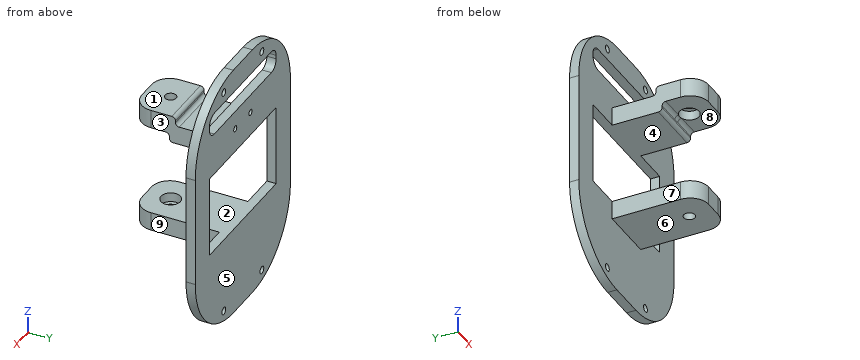
```python
from build123d import *

# Parameters (mm, degrees)
SKETCH1_W           = 100
SKETCH1_H           = 90
BOSS_EXTRUDE1_DEPTH = 5
SKETCH2_W           = 70
SKETCH2_H           = 44
CUT_EXTRUDE1_DEPTH  = 68.453687816
SKETCH3_R           = 1.6
CUT_EXTRUDE2_DEPTH  = 68.453687816
SKETCH4_W           = 100
SKETCH4_H           = 25
BOSS_EXTRUDE2_DEPTH = 5
SKETCH6_W           = 70
SKETCH6_H           = 12
CUT_EXTRUDE4_DEPTH  = 17
SKETCH8_W           = 30
SKETCH8_H           = 10
BOSS_EXTRUDE4_DEPTH = 47
SKETCH11_R          = 5.25
CUT_EXTRUDE5_DEPTH  = 5
SKETCH12_R          = 3
CUT_EXTRUDE6_DEPTH  = 5
FILLET1_R           = 10
CUT_EXTRUDE7_START  = -5
SKETCH13_R          = 5.25
CUT_EXTRUDE7_DEPTH  = 5
CUT_EXTRUDE8_START  = -5
SKETCH14_R          = 3
CUT_EXTRUDE8_DEPTH  = 5
FILLET2_R           = 10
SKETCH15_R          = 2
CUT_EXTRUDE9_DEPTH  = 101.518654985
FILLET3_R           = 40
FILLET4_R           = 40
FILLET5_R           = 5
BOSS_EXTRUDE5_DEPTH = 30
SKETCH17_R          = 5.25
CUT_EXTRUDE10_DEPTH = 10
SKETCH18_R          = 3
CUT_EXTRUDE12_DEPTH = 21
CUT_EXTRUDE13_DEPTH = 21
SKETCH20_W          = 5
SKETCH20_H          = 20
CUT_EXTRUDE14_DEPTH = 107.46126056
FILLET6_R           = 2
FILLET7_R           = 2


with BuildPart() as part:
    # Sketch1 → Boss-Extrude1 (new body)
    with BuildSketch(Plane(origin=(0, 0, 0), x_dir=(1, 0, 0), z_dir=(0, 1, 0))):
        Rectangle(SKETCH1_W, SKETCH1_H)
    extrude(amount=BOSS_EXTRUDE1_DEPTH)

    # Sketch2 → Cut-Extrude1 (cut, through all)
    with BuildSketch(Plane(origin=(0, 5, 0), x_dir=(1, 0, 0), z_dir=(0, 1, 0))):
        Rectangle(SKETCH2_W, SKETCH2_H)
    extrude(amount=-CUT_EXTRUDE1_DEPTH, mode=Mode.SUBTRACT)

    # Sketch3 → Cut-Extrude2 (cut, through all)
    with BuildSketch(Plane(origin=(0, 5, 0), x_dir=(1, 0, 0), z_dir=(0, 1, 0))):
        with Locations(Location((-8, -35, 0), (0, 0, 270))):
            Circle(SKETCH3_R)
        with Locations(Location((8, -35, 0), (0, 0, 90))):
            Circle(SKETCH3_R)
    extrude(amount=-CUT_EXTRUDE2_DEPTH, mode=Mode.SUBTRACT)

    # Sketch4 → Boss-Extrude2 (add)
    with BuildSketch(Plane(origin=(0, 5, 0), x_dir=(1, 0, 0), z_dir=(0, 1, 0))):
        with Locations((0, -57.5)):
            Rectangle(SKETCH4_W, SKETCH4_H)
        with Locations((0, 57.5)):
            Rectangle(SKETCH4_W, SKETCH4_H)
    extrude(amount=-BOSS_EXTRUDE2_DEPTH)

    # Sketch6 → Cut-Extrude4 (cut)
    with BuildSketch(Plane(origin=(0, 5, 0), x_dir=(1, 0, 0), z_dir=(0, 1, 0))):
        with Locations((0, -51)):
            Rectangle(SKETCH6_W, SKETCH6_H)
    extrude(amount=-CUT_EXTRUDE4_DEPTH, mode=Mode.SUBTRACT)

    # Sketch8 → Boss-Extrude4 (add)
    with BuildSketch(Plane.XZ):
        with Locations((0, 27)):
            Rectangle(SKETCH8_W, SKETCH8_H)
        with Locations((0, -27)):
            Rectangle(SKETCH8_W, SKETCH8_H)
    extrude(amount=BOSS_EXTRUDE4_DEPTH)

    # Sketch11 → Cut-Extrude5 (cut)
    with BuildSketch(Plane(origin=(0, 0, 22), x_dir=(-1, 0, 0), z_dir=(0, 0, -1))):
        with Locations((0, -34)):
            Circle(SKETCH11_R)
    extrude(amount=-CUT_EXTRUDE5_DEPTH, mode=Mode.SUBTRACT)

    # Sketch12 → Cut-Extrude6 (cut)
    with BuildSketch(Plane(origin=(0, 0, 27), x_dir=(-1, 0, 0), z_dir=(0, 0, -1))):
        with Locations((0, -34)):
            Circle(SKETCH12_R)
    extrude(amount=-CUT_EXTRUDE6_DEPTH, mode=Mode.SUBTRACT)

    # Fillet1
    fillet1_edges = [part.edges().sort_by_distance(p)[0] for p in [
        (-15, -47, 27),
        (15, -47, 27),
    ]]
    fillet(fillet1_edges, radius=FILLET1_R)

    # Sketch13 → Cut-Extrude7 (cut)
    with BuildSketch(Plane.XY.offset(-22).offset(CUT_EXTRUDE7_START)):
        with Locations(Location((0, -34, 0), (0, 0, 180))):
            Circle(SKETCH13_R)
    extrude(amount=CUT_EXTRUDE7_DEPTH, mode=Mode.SUBTRACT)

    # Sketch14 → Cut-Extrude8 (cut)
    with BuildSketch(Plane.XY.offset(-27).offset(CUT_EXTRUDE8_START)):
        with Locations(Location((0, -34, 0), (0, 0, 180))):
            Circle(SKETCH14_R)
    extrude(amount=CUT_EXTRUDE8_DEPTH, mode=Mode.SUBTRACT)

    # Fillet2
    fillet2_edges = [part.edges().sort_by_distance(p)[0] for p in [
        (15, -47, -27),
        (-15, -47, -27),
    ]]
    fillet(fillet2_edges, radius=FILLET2_R)

    # Sketch15 → Cut-Extrude9 (cut, through all)
    with BuildSketch(Plane(origin=(0, 5, 0), x_dir=(1, 0, 0), z_dir=(0, 1, 0))):
        with Locations(Location((-20, -63, 0), (0, 0, 270))):
            Circle(SKETCH15_R)
        with Locations(Location((-20, 63, 0), (0, 0, 270))):
            Circle(SKETCH15_R)
        with Locations(Location((20, -63, 0), (0, 0, 270))):
            Circle(SKETCH15_R)
        with Locations(Location((20, 63, 0), (0, 0, 270))):
            Circle(SKETCH15_R)
    extrude(amount=-CUT_EXTRUDE9_DEPTH, mode=Mode.SUBTRACT)

    # Fillet3
    fillet3_edges = [part.edges().sort_by_distance(p)[0] for p in [
        (-50, 2.5, 70),
        (50, 2.5, 70),
    ]]
    fillet(fillet3_edges, radius=FILLET3_R)

    # Fillet4
    fillet4_edges = [part.edges().sort_by_distance(p)[0] for p in [
        (-50, 2.5, -70),
        (50, 2.5, -70),
    ]]
    fillet(fillet4_edges, radius=FILLET4_R)

    # Fillet5
    fillet5_edges = [part.edges().sort_by_distance(p)[0] for p in [
        (-35, 2.5, 57),
        (-35, 2.5, 45),
        (35, 2.5, 45),
        (35, 2.5, 57),
    ]]
    fillet(fillet5_edges, radius=FILLET5_R)

    # Sketch16 → Boss-Extrude5 (add)
    with BuildSketch(Plane(origin=(15, 0, 0), x_dir=(0, 0, -1), z_dir=(1, 0, 0))):
        Polygon((-32, -23.652392467), (-37, -23.652392467), (-37, -47), (-27, -47), (-27, -23.652392467), align=None)
    extrude(amount=-BOSS_EXTRUDE5_DEPTH)

    # Sketch17 → Cut-Extrude10 (cut)
    with BuildSketch(Plane(origin=(0, 0, 22), x_dir=(-1, 0, 0), z_dir=(0, 0, -1))):
        with Locations((0, -34)):
            Circle(SKETCH17_R)
    extrude(amount=-CUT_EXTRUDE10_DEPTH, mode=Mode.SUBTRACT)

    # Sketch18 → Cut-Extrude12 (cut)
    with BuildSketch(Plane(origin=(0, 0, 22), x_dir=(-1, 0, 0), z_dir=(0, 0, -1))):
        with Locations(Location((0, -34, 0), (0, 0, 180))):
            Circle(SKETCH18_R)
    extrude(amount=-CUT_EXTRUDE12_DEPTH, mode=Mode.SUBTRACT)

    # Sketch19 → Cut-Extrude13 (cut)
    with BuildSketch(Plane(origin=(0, 0, 22), x_dir=(-1, 0, 0), z_dir=(0, 0, -1))):
        with BuildLine():
            Line((-15, -37), (-15, -47))
            Line((-15, -47), (-5, -47))
            ThreePointArc((-5, -47), (-12.071067812, -44.071067812), (-15, -37))
        make_face()
        with BuildLine():
            Line((5, -47), (15, -47))
            Line((15, -47), (15, -37))
            ThreePointArc((15, -37), (12.071067812, -44.071067812), (5, -47))
        make_face()
    extrude(amount=-CUT_EXTRUDE13_DEPTH, mode=Mode.SUBTRACT)

    # Sketch20 → Cut-Extrude14 (cut, through all)
    with BuildSketch(Plane(origin=(15, 0, 0), x_dir=(0, 0, -1), z_dir=(1, 0, 0))):
        with Locations((-24.5, -37)):
            Rectangle(SKETCH20_W, SKETCH20_H)
    extrude(amount=-CUT_EXTRUDE14_DEPTH, mode=Mode.SUBTRACT)

    # Fillet6
    fillet6_edges = [part.edges().sort_by_distance(p)[0] for p in [
        (0, -23.652392467, 32),
        (0, -23.652392467, 37),
    ]]
    fillet(fillet6_edges, radius=FILLET6_R)

    # Fillet7
    fillet7_edges = [part.edges().sort_by_distance(p)[0] for p in [
        (0, -27, 27),
        (0, -27, 22),
    ]]
    fillet(fillet7_edges, radius=FILLET7_R)


solid = part.part
```
Work out the finished part from the listing and answer in its coordinate system (mm). Face numbers are marked on the shaded views. A direction names the side the tool comes from. Give positions to 0.01 mm unless a question says otherwise; leave off trailing zeros. Loops run counter-clockwise (first coordinate to the right, second up) from the corner with the lowest first, then second, coordinate; pieces in that order, holes last. Notation, with made-up numbers: (-17.5, 53.5) -> (-6.5, 53.5) arc R19 cw to (-6.5, 88.5) -> close; hole circle Ø4 at (51, -8). An arc over 180 degrees is marked (long way). One line per question, with ' | ' between items. Start each with the question number.
1) For the marked faces 5, 6, 7, 8 and 9, determine the directions among +Z, -Z, +X, -X, +Y, -Y from which every point of the face is accessible in a straight line to the end or side of a thin tool.
2) Section D-D, the plane y = -12 is taken. Determine the outline of the cut face in (x, z), then the cut area to 3 significant figures.
3) Determine the mould class of the marked faces 1, 2, 3 and 4 for opening direction Z: +Z half, -Z half, draft (parallel to the pull), parting line (faces both ways), or undercut.
4) Straight lines are drawn through the part: L1, parallel to Z at x = -1.5, y = -14; L2, parallel to X at y = -34, z = -25; L3, parallel to X at y = -34, z = 35. For each, find the intervals that lie inside material, in ascending order.
5) Each of these flat-tipped pins is pushed along its axis until it touches: pin 1 (12 mm diameter, centred on x = 21.5, z = 44.5, fed in from -Y); pin 2 (14.5 mm diameter, centred on x = -1.5, y = -35, fed in from -Z); pin 3 (23.5 mm diameter, centred on x = -2, y = -34.5, fed in from +Z). Where does it stop, or does it pass through?
6) Section B-B, the plane y = -34 is taken. Determine the outline of the cut face in (x, z), then the cut area to 3 significant figures.
7) Section C-C, the plane x = 20 is taken. Determine the outline of the cut face in (y, z).
8) Section A-A, the plane z = 19.5 is taken. Determine the outline of the cut face in (x, y), then the cut area to 3 significant figures.
Resolved:
1) face 5: +Z, -Z, +X, -X, +Y | face 6: -Z, +X, -X, -Y | face 7: +Z, -Z, -X, -Y | face 8: +X, -X, -Y | face 9: +Z, -Z, +X, -Y
2) outline: (-15, -32) -> (15, -32) -> (15, -22) -> (-15, -22) -> close; (-15, 22) -> (15, 22) -> (15, 32) -> (-15, 32) -> close | area: 600 mm2
3) face 1: +Z half | face 2: undercut | face 3: draft | face 4: undercut
4) L1: -32 to -22, 22 to 32 | L2: -15 to -5.25, 5.25 to 15 | L3: -15 to -3, 3 to 15
5) pin 1: y = 0 | pin 2: z = -32 | pin 3: z = 37
6) outline: (-15, -32) -> (-3, -32) -> (-3, -27) -> (-5.25, -27) -> (-5.25, -22) -> (-15, -22) -> close; (-15, 27) -> (-5.25, 27) -> (-5.25, 32) -> (-3, 32) -> (-3, 37) -> (-15, 37) -> close; (3, -32) -> (15, -32) -> (15, -22) -> (5.25, -22) -> (5.25, -27) -> (3, -27) -> close; (3, 32) -> (5.25, 32) -> (5.25, 27) -> (15, 27) -> (15, 37) -> (3, 37) -> close | area: 435 mm2
7) outline: (0, -68.73) -> (5, -68.73) -> (5, -65) -> (0, -65) -> close; (0, -61) -> (5, -61) -> (5, -22) -> (0, -22) -> close; (0, 22) -> (5, 22) -> (5, 45) -> (0, 45) -> close; (0, 57) -> (5, 57) -> (5, 61) -> (0, 61) -> close; (0, 65) -> (5, 65) -> (5, 68.73) -> (0, 68.73) -> close
8) outline: (-50, 0) -> (-35, 0) -> (-35, 5) -> (-50, 5) -> close; (35, 0) -> (50, 0) -> (50, 5) -> (35, 5) -> close | area: 150 mm2
